```python
from build123d import *

# Parameters (mm, degrees)
SKETCH1_W                      = 26.2
SKETCH1_H                      = 7.2
BOSS_EXTRUDE1_DEPTH            = 6.95
SKETCH2_W                      = 5
SKETCH2_H                      = 0.7
CUT_EXTRUDE1_DEPTH             = 24.916991868
CUT_EXTRUDE2_DEPTH             = 25.716441896
CUT_EXTRUDE3_DEPTH             = 25.716441896
SKETCH5_W                      = 13.4
SKETCH5_H                      = 6.2
BOSS_EXTRUDE2_DEPTH            = 7.55
SKETCH6_W                      = 13
SKETCH6_H                      = 0.7
BOSS_EXTRUDE3_DEPTH            = 3.8
SKETCH7_W                      = 1.5
SKETCH7_H                      = 0.3
BOSS_EXTRUDE4_DEPTH            = 6.2
SKETCH8_W                      = 1.5
SKETCH8_H                      = 0.3
BOSS_EXTRUDE5_DEPTH            = 6.2
SKETCH9_W                      = 1.5
SKETCH9_H                      = 0.3
BOSS_EXTRUDE6_DEPTH            = 6.2
SKETCH10_W                     = 2.5
SKETCH10_H                     = 0.3
BOSS_EXTRUDE7_DEPTH            = 6.2
SKETCH11_W                     = 3.2
SKETCH11_H                     = 3.2
CUT_EXTRUDE4_DEPTH             = 1
SKETCH12_W                     = 3
SKETCH12_H                     = 3
BOSS_EXTRUDE8_DEPTH            = 1
SKETCH13_W                     = 4.2
SKETCH13_H                     = 6.35
BOSS_EXTRUDE9_DEPTH            = 8.3
SKETCH14_W                     = 0.8
SKETCH14_H                     = 2
CUT_EXTRUDE5_DEPTH             = 0.2
SKETCH15_W                     = 4.2
SKETCH15_H                     = 6.35
BOSS_EXTRUDE10_DEPTH           = 8.3
SKETCH16_W                     = 0.8
SKETCH16_H                     = 2
CUT_EXTRUDE6_DEPTH             = 0.2
F_3_2_3_2_DIAMETER_HOLE1_D     = 3.2
F_3_2_3_2_DIAMETER_HOLE1_DEPTH = 1.875
F_3_2_3_2_DIAMETER_HOLE2_D     = 3.2
F_3_2_3_2_DIAMETER_HOLE2_DEPTH = 6.95


with BuildPart() as part:
    # Sketch1 → Boss-Extrude1 (new body)
    with BuildSketch(Plane.XY.offset(6.95)):
        with Locations((9.5, 0)):
            Rectangle(SKETCH1_W, SKETCH1_H)
    extrude(amount=-BOSS_EXTRUDE1_DEPTH)

    # Sketch2 → Cut-Extrude1 (cut, through all)
    with BuildSketch(Plane(origin=(0, 0, 0), x_dir=(-1, 0, 0), z_dir=(0, 0, -1))):
        with Locations((-9.5, 3.25)):
            Rectangle(SKETCH2_W, SKETCH2_H)
    extrude(amount=-CUT_EXTRUDE1_DEPTH, mode=Mode.SUBTRACT)

    # Sketch3 → Cut-Extrude2 (cut, through all)
    with BuildSketch(Plane.XZ.offset(3.6)):
        with BuildLine():
            Line((1.612876483, 5.075), (-1.612876483, 5.075))
            ThreePointArc((-1.612876483, 5.075), (-2, 3.475), (-1.612876483, 1.875))
            Line((-1.612876483, 1.875), (1.612876483, 1.875))
            ThreePointArc((1.612876483, 1.875), (2, 3.475), (1.612876483, 5.075))
        make_face()
    extrude(amount=-CUT_EXTRUDE2_DEPTH, mode=Mode.SUBTRACT)

    # Sketch4 → Cut-Extrude3 (cut, through all)
    with BuildSketch(Plane.XZ.offset(3.6)):
        with BuildLine():
            Line((17.387123517, 1.875), (20.612876483, 1.875))
            ThreePointArc((20.612876483, 1.875), (21, 3.475), (20.612876483, 5.075))
            Line((20.612876483, 5.075), (17.387123517, 5.075))
            ThreePointArc((17.387123517, 5.075), (17, 3.475), (17.387123517, 1.875))
        make_face()
    extrude(amount=-CUT_EXTRUDE3_DEPTH, mode=Mode.SUBTRACT)

    # Sketch5 → Boss-Extrude2 (add)
    with BuildSketch(Plane.XY.offset(6.95)):
        with Locations((9.5, -0.5)):
            Rectangle(SKETCH5_W, SKETCH5_H)
    extrude(amount=BOSS_EXTRUDE2_DEPTH)

    # Sketch6 → Boss-Extrude3 (add)
    with BuildSketch(Plane.XY.offset(14.5)):
        with Locations((9.5, -2.65)):
            Rectangle(SKETCH6_W, SKETCH6_H)
    extrude(amount=BOSS_EXTRUDE3_DEPTH)

    # Sketch7 → Boss-Extrude4 (add)
    with BuildSketch(Plane.XY.offset(14.5)):
        with Locations((13.31, -0.2)):
            Rectangle(SKETCH7_W, SKETCH7_H)
    extrude(amount=BOSS_EXTRUDE4_DEPTH)

    # Sketch8 → Boss-Extrude5 (add)
    with BuildSketch(Plane.XY.offset(14.5)):
        with Locations((10.77, -0.2)):
            Rectangle(SKETCH8_W, SKETCH8_H)
    extrude(amount=BOSS_EXTRUDE5_DEPTH)

    # Sketch9 → Boss-Extrude6 (add)
    with BuildSketch(Plane.XY.offset(14.5)):
        with Locations((8.23, -0.2)):
            Rectangle(SKETCH9_W, SKETCH9_H)
    extrude(amount=BOSS_EXTRUDE6_DEPTH)

    # Sketch10 → Boss-Extrude7 (add)
    with BuildSketch(Plane.XY.offset(14.5)):
        with Locations((5.19, -0.2)):
            Rectangle(SKETCH10_W, SKETCH10_H)
    extrude(amount=BOSS_EXTRUDE7_DEPTH)

    # Sketch11 → Cut-Extrude4 (cut)
    with BuildSketch(Plane(origin=(0, 2.6, 0), x_dir=(-1, 0, 0), z_dir=(0, 1, 0))):
        with Locations((-8, 8.8)):
            Rectangle(SKETCH11_W, SKETCH11_H)
    extrude(amount=-CUT_EXTRUDE4_DEPTH, mode=Mode.SUBTRACT)

    # Sketch12 → Boss-Extrude8 (add)
    with BuildSketch(Plane(origin=(0, 1.6, 0), x_dir=(-1, 0, 0), z_dir=(0, 1, 0))):
        with Locations((-8, 8.8)):
            Rectangle(SKETCH12_W, SKETCH12_H)
    extrude(amount=BOSS_EXTRUDE8_DEPTH)

    # Sketch13 → Boss-Extrude9 (add)
    with BuildSketch(Plane(origin=(0, 3.6, 0), x_dir=(-1, 0, 0), z_dir=(0, 1, 0))):
        with Locations((-14.1, 3.475)):
            Rectangle(SKETCH13_W, SKETCH13_H)
    extrude(amount=BOSS_EXTRUDE9_DEPTH)

    # Sketch14 → Cut-Extrude5 (cut)
    with BuildSketch(Plane.ZY.offset(-12)):
        with Locations((3.475, 9)):
            Rectangle(SKETCH14_W, SKETCH14_H)
    extrude(amount=-CUT_EXTRUDE5_DEPTH, mode=Mode.SUBTRACT)

    # Sketch15 → Boss-Extrude10 (add)
    with BuildSketch(Plane(origin=(0, 3.6, 0), x_dir=(-1, 0, 0), z_dir=(0, 1, 0))):
        with Locations((-4.9, 3.475)):
            Rectangle(SKETCH15_W, SKETCH15_H)
    extrude(amount=BOSS_EXTRUDE10_DEPTH)

    # Sketch16 → Cut-Extrude6 (cut)
    with BuildSketch(Plane(origin=(7, 0, 0), x_dir=(0, 0, -1), z_dir=(1, 0, 0))):
        with Locations((-3.475, 9)):
            Rectangle(SKETCH16_W, SKETCH16_H)
    extrude(amount=-CUT_EXTRUDE6_DEPTH, mode=Mode.SUBTRACT)

    # Ø3.2 (3.2) Diameter Hole1
    with Locations(Plane(origin=(0, 0, 0), x_dir=(-1, 0, 0), z_dir=(0, 0, -1))):
        with Locations((0, 0), (-19, 0)):
            Hole(F_3_2_3_2_DIAMETER_HOLE1_D / 2, depth=F_3_2_3_2_DIAMETER_HOLE1_DEPTH)

    # Ø3.2 (3.2) Diameter Hole2
    with Locations(Plane.XY.offset(6.95)):
        with Locations((19, 0), (0, 0)):
            Hole(F_3_2_3_2_DIAMETER_HOLE2_D / 2, depth=F_3_2_3_2_DIAMETER_HOLE2_DEPTH)


solid = part.part
```
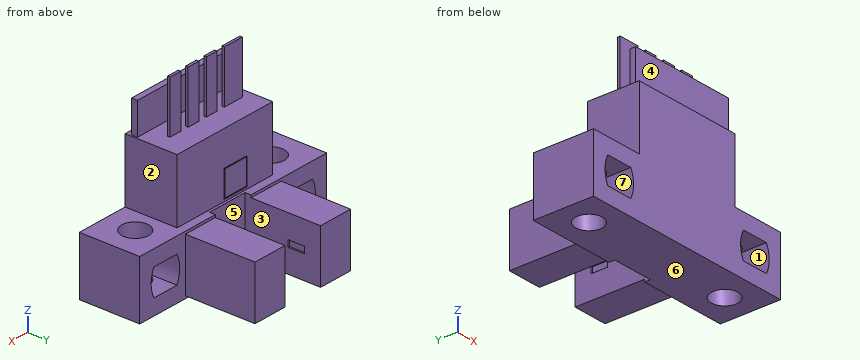
Model file for the job. Use its own axes, mm. Face numbers are marked on the shaded views. A direction names the side the tool comes from. Coordinates: 2 decimals unless noted, no trailing zeros. Loops run counter-clockwise (first coordinate to the right, second up) from the corner with the lowest first, then second, coordinate; pieces in that order, holes last. Notation, with made-up numbers: M -4.75,18 L 26.25,18 A20 cw 26.25,41 Z; hole C 44.25,55 d2. An arc over 180 degrees is marked long. Use CSV: the item, a comma, the result in double quotes. Start each with the question number.
1. Band-saw the part on D-D, the plane z = 4.75. List the corners of the cut face in (x, y), then the cut area to 3 significant figures.
2. Band-saw the part on A-A, the plane z = 16.25. List the corners of the cut face in (x, y), then the cut area to 3 significant figures.
3. Probe probe 1 along X at (y, z) = (0, 1.2); probe 2 along Y at (x, z) = (0, 0.7); probe 3 along X at (y, z) = (6.75, 5.5). List the from-to ranges inside material, lowest first. Write a range as [from, to].
4. Band-saw the part on C-C, the plane x = 0. List the corners of the cut face in (y, z) (3 decimals), then the cut area to 3 significant figures.
5. Band-saw the part on B-B, the plane y = 9. List the corners of the cut face in (x, z) (3 decimals).
6. Tool access for the marked faces 1, 2, 3 and 4: list every direction of +Z, -Z, +X, -X, +Y, -Y with a clear straight run to the whole face (end or side of a thin tool).
7. Flat gauge pins, fed straight in: pin 1 (1 mm diameter, centred on x = 2, y = 1.5, fed in from +Z); pin 2 (0.9 mm diameter, centred on x = 8, z = 9.5, fed in from +Y); pin 3 (1.1 mm diameter, centred on x = 7.5, y = 2, fed in from +Z); pin 4 (2.5 mm diameter, centred on x = 0, y = 0, fed in from +Z). Where does each tip first touch, or does it go through?
8. Two-plate mould, pull along Z, no slides. Class the marked faces 5, 6 and 7: pulls with the +Z half, pulls with the -Z half, needs draft (parallel to the pull), parting line crosses it, or undercut.
Entries:
1,outline,"M -3.6,-3.6 L -1.76,-3.6 L -1.76,3.6 L -3.6,3.6 Z; M 1.76,-3.6 L 17.24,-3.6 L 17.24,3.6 L 16.2,3.6 L 16.2,11.9 L 12,11.9 L 12,2.9 L 7,2.9 L 7,11.9 L 2.8,11.9 L 2.8,3.6 L 1.76,3.6 Z; M 20.76,-3.6 L 22.6,-3.6 L 22.6,3.6 L 20.76,3.6 Z"
1,area,"204 mm2"
2,outline,"M 3,-3 L 16,-3 L 16,-2.3 L 3,-2.3 Z; M 3.94,-0.35 L 6.44,-0.35 L 6.44,-0.05 L 3.94,-0.05 Z; M 7.48,-0.35 L 8.98,-0.35 L 8.98,-0.05 L 7.48,-0.05 Z; M 10.02,-0.35 L 11.52,-0.35 L 11.52,-0.05 L 10.02,-0.05 Z; M 12.56,-0.35 L 14.06,-0.35 L 14.06,-0.05 L 12.56,-0.05 Z"
2,area,"11.2 mm2"
3,probe 1,"x = [-3.6, -1.6], [1.6, 17.4], [20.6, 22.6]"
3,probe 2,"y = [-3.6, -1.6], [1.6, 3.6]"
3,probe 3,"x = [2.8, 7], [12, 16.2]"
4,outline,"M -3.6,0 L -1.6,0 L -1.6,1.875 L -3.6,1.875 Z; M -3.6,5.075 L -1.6,5.075 L -1.6,6.95 L -3.6,6.95 Z; M 1.6,0 L 3.6,0 L 3.6,1.875 L 1.6,1.875 Z; M 1.6,5.075 L 3.6,5.075 L 3.6,6.95 L 1.6,6.95 Z"
4,area,"15.0 mm2"
5,outline,"M 2.8,0.3 L 7,0.3 L 7,3.075 L 6.8,3.075 L 6.8,3.875 L 7,3.875 L 7,6.65 L 2.8,6.65 Z; M 12,0.3 L 16.2,0.3 L 16.2,6.65 L 12,6.65 L 12,3.875 L 12.2,3.875 L 12.2,3.075 L 12,3.075 Z"
6,face 1,"+Y, -Y"
6,face 2,"+Z, +X, +Y, -Y"
6,face 3,"+Z, -Z, +Y"
6,face 4,"+Z, +X, -X, -Y"
7,pin 1,"stops at z = 6.95"
7,pin 2,"stops at y = 2.6"
7,pin 3,"stops at z = 14.5"
7,pin 4,"passes through"
8,face 5,"needs draft"
8,face 6,"pulls with the -Z half"
8,face 7,"undercut"
